Geometry: see drawing. Coordinates: mm, zero at the bounding-box minimum. Round coordinates to 2 decimals unless told otherwise and drop trailing zeros. Loops run counter-clockwise (first coordinate to the right, second up) from the corner with the lowest first, then second, coordinate; pieces in that order, holes last. Notation, with made-up numbers: (59, 75) -> (71, 75) arc R25 cw to (71, 92) -> close; hole circle Ø11 at (60, -26). An arc over 180 degrees is marked (long way). Answer in a Markdown table with one row per item.
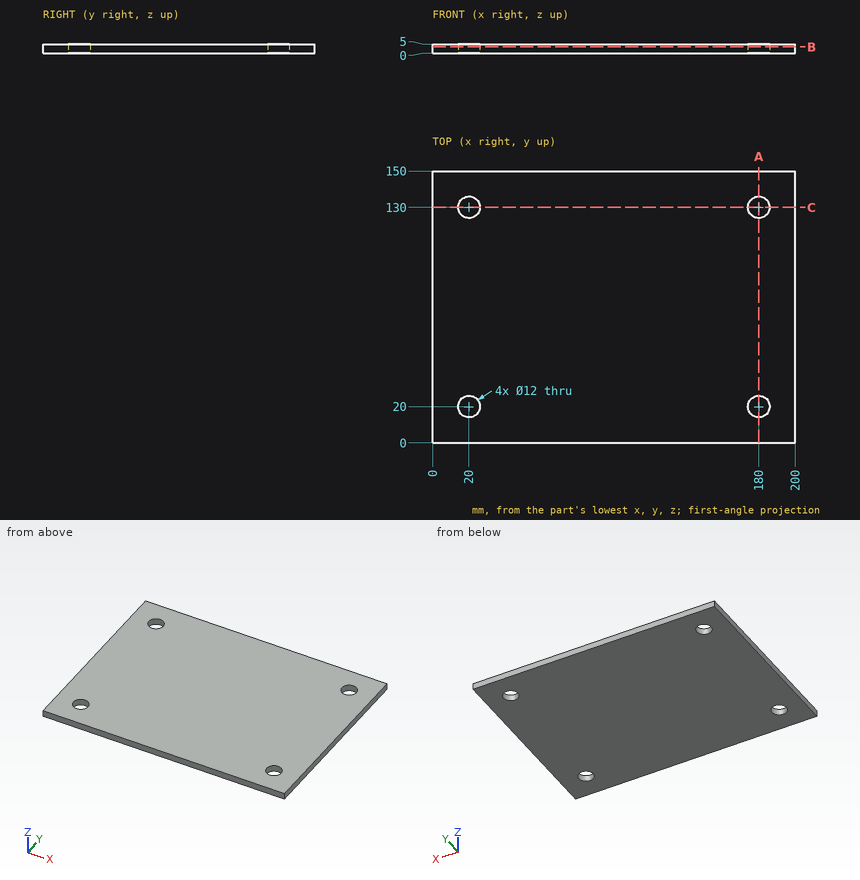
Item 1: Section query B-B, the plane z = 3.45. Output: boundary loops of the cut face in (x, y), and give its area (3 significant figures).
Ans:
| item | result |
|---|---|
| outline | (0, 0) -> (200, 0) -> (200, 150) -> (0, 150) -> close; hole circle Ø12 at (20, 20); hole circle Ø12 at (20, 130); hole circle Ø12 at (180, 20); hole circle Ø12 at (180, 130) |
| area | 29,500 mm2 |
Item 2: First-contact query: P1, Ø8, axis at x = 34.5, y = 128, coming from the -Z side. Flat tip, straight axial feed; report the tip coordinate or a pass-through.
Ans:
| item | result |
|---|---|
| P1 | z = 0 |
Item 3: Ray query, L1, parallel to Y at x = 180, z = 3.3; L2, parallel to X at y = 23, z = 2.65. Return the intervals inside material, ascending.
Ans:
| item | result |
|---|---|
| L1 | 0 to 14, 26 to 124, 136 to 150 |
| L2 | 0 to 14.8, 25.2 to 174.8, 185.2 to 200 |
Item 4: Section query C-C, the plane y = 130. Output: boundary loops of the cut face in (x, z).
Ans:
| item | result |
|---|---|
| outline | (0, 0) -> (14, 0) -> (14, 5) -> (0, 5) -> close; (26, 0) -> (174, 0) -> (174, 5) -> (26, 5) -> close; (186, 0) -> (200, 0) -> (200, 5) -> (186, 5) -> close |
Item 5: Section query A-A, the plane x = 180. Output: boundary loops of the cut face in (y, z), and give its area (3 significant figures).
Ans:
| item | result |
|---|---|
| outline | (0, 0) -> (14, 0) -> (14, 5) -> (0, 5) -> close; (26, 0) -> (124, 0) -> (124, 5) -> (26, 5) -> close; (136, 0) -> (150, 0) -> (150, 5) -> (136, 5) -> close |
| area | 630 mm2 |
